Work out the finished part from the listing and answer in its coordinate system (mm). A direction names the side the tool comes from. Coordinates: 2 decimals unless noted, no trailing zeros. Order: outer loops, then holes, each group sorted by start corner. A loop starts at its lowest first (then second) coordinate and runs counter-clockwise, first axis right, second up.
1. The part is cut by section B-B, the plane y = 61.5. Give the vertices of the cut face in (x, z), then the cut area to 4 significant figures.
2. Determine the mould class of faces 1 (the cylindrical face through (-79.446, -137.712, 2.465)), 2 (the cylindrical face through (123.956, 0.266, 2.465)), 3 (the cylindrical face through (146.99, 97.15, 2.54)) for opening direction Y: +Y half, -Y half, draft (parallel to the pull), parting line (faces both ways), or undercut.
3. Flat-ended cylindrical pins translate along their axes: pin 1 Ø5 at (x, y) = (192.5, -100) entering from +Z; pin 2 Ø1 at (y, z) = (-7, 2.5) entering from -X; pin 3 Ø2 at (x, z) = (143.5, 2) entering from +Y. Find the tip coordinate at first contact, or state that the pin passes through.
4. The part is cut by section D-D, the plane z = 1.4. Count the separate pieces of the cut face and the enclosed holes in it, then the cut area to 3 significant figures.
5. The part is cut by section A-A, the plane x = 50. Give the vertices of the cut face in (y, z), then the cut area to 4 significant figures.
6. The part is cut by section C-C, the plane x = 130. Give the vertices of the cut face in (y, z).
7. Find the intervals of material crossed by probe 1 along Y at (x, z) = (14, 2.65); probe 2 along Y at (x, z) = (178.5, 0.8); probe 3 along X at (y, z) = (-73.5, 4.75), in increasing order.
8. A tool of negligible diameter and unlimited length cuts with its end or side. For faces 4 (the cylindrical face through (-147.15, 96.99, 2.54)), 5 (the cylindrical face through (79.055, -136.97, 2.465)), 6 (the flat face through (-78, -44, 3)), from which of +Z, -Z, +X, -X, +Y, -Y can it reach the whole face along a straight path? Write none if from no direction.
```python
from build123d import *

# Parameters (mm, degrees)
EXTRUDE_1_OUTLINE_R   = 2
EXTRUDE_1_OUTLINE_R_2 = 6.05
EXTRUDE_1_DEPTH       = 5
CUT_EXTRUDE_START     = -2
SKETCH_2_R            = 3
SKETCH_2_R_2          = 2
CUT_EXTRUDE_1_DEPTH   = 2
SKETCH_3_R            = 31
SKETCH_3_R_2          = 32
CUT_EXTRUDE_2_DEPTH   = 281.579587951
FILLET_1_R            = 10
SKETCH1_R             = 11.937888281
CUT_EXTRUDE1_DEPTH    = 10
FILLET1_R             = 5


# Read off the part's stored shape, not the designer's step: 凸台-拉伸1
with BuildPart() as part:
    # 凸台-拉伸1 outline → 凸台-拉伸1 (new body)
    with BuildSketch(Plane.XY):
        with BuildLine():
            ThreePointArc((-97.800454043, -160.623488863), (-77.281489026, -133.346936317), (-70, -100))
            Line((-70, -100), (70, -100))
            ThreePointArc((70, -100), (77.281489026, -133.346936317), (97.800454043, -160.623488863))
            Line((97.800454043, -160.623488863), (202.199545957, -160.623488863))
            ThreePointArc((202.199545957, -160.623488863), (224.999597029, -72.160092574), (150, -20))
            Line((150, -20), (150, 100))
            Line((150, 100), (-150, 100))
            Line((-150, 100), (-150, -20))
            ThreePointArc((-150, -20), (-224.999597029, -72.160092574), (-202.199545957, -160.623488863))
            Line((-202.199545957, -160.623488863), (-97.800454043, -160.623488863))
        make_face()
        with Locations((-180.0520382, -130.0520382)):
            Circle(EXTRUDE_1_OUTLINE_R, mode=Mode.SUBTRACT)
        with Locations((-150, -142.5)):
            Circle(EXTRUDE_1_OUTLINE_R, mode=Mode.SUBTRACT)
        with Locations((-119.9479618, -130.0520382)):
            Circle(EXTRUDE_1_OUTLINE_R, mode=Mode.SUBTRACT)
        with Locations((-192.5, -100)):
            Circle(EXTRUDE_1_OUTLINE_R, mode=Mode.SUBTRACT)
        with Locations((-107.5, -100)):
            Circle(EXTRUDE_1_OUTLINE_R, mode=Mode.SUBTRACT)
        with Locations((-180.0520382, -69.9479618)):
            Circle(EXTRUDE_1_OUTLINE_R, mode=Mode.SUBTRACT)
        with Locations((-119.9479618, -69.9479618)):
            Circle(EXTRUDE_1_OUTLINE_R, mode=Mode.SUBTRACT)
        with Locations((-150, -57.5)):
            Circle(EXTRUDE_1_OUTLINE_R, mode=Mode.SUBTRACT)
        with Locations((-50, -80)):
            Circle(EXTRUDE_1_OUTLINE_R_2, mode=Mode.SUBTRACT)
        with Locations((107.5, -100)):
            Circle(EXTRUDE_1_OUTLINE_R, mode=Mode.SUBTRACT)
        with Locations((119.9479618, -130.0520382)):
            Circle(EXTRUDE_1_OUTLINE_R, mode=Mode.SUBTRACT)
        with Locations((150, -142.5)):
            Circle(EXTRUDE_1_OUTLINE_R, mode=Mode.SUBTRACT)
        with Locations((180.0520382, -130.0520382)):
            Circle(EXTRUDE_1_OUTLINE_R, mode=Mode.SUBTRACT)
        with Locations((192.5, -100)):
            Circle(EXTRUDE_1_OUTLINE_R, mode=Mode.SUBTRACT)
        with Locations((50, -80)):
            Circle(EXTRUDE_1_OUTLINE_R_2, mode=Mode.SUBTRACT)
        with Locations((119.9479618, -69.9479618)):
            Circle(EXTRUDE_1_OUTLINE_R, mode=Mode.SUBTRACT)
        with Locations((180.0520382, -69.9479618)):
            Circle(EXTRUDE_1_OUTLINE_R, mode=Mode.SUBTRACT)
        with Locations((150, -57.5)):
            Circle(EXTRUDE_1_OUTLINE_R, mode=Mode.SUBTRACT)
        with Locations((-130, 0)):
            Circle(EXTRUDE_1_OUTLINE_R_2, mode=Mode.SUBTRACT)
        with Locations((-130, 79.62392947)):
            Circle(EXTRUDE_1_OUTLINE_R_2, mode=Mode.SUBTRACT)
        with Locations((130, 0)):
            Circle(EXTRUDE_1_OUTLINE_R_2, mode=Mode.SUBTRACT)
        with Locations((130, 80)):
            Circle(EXTRUDE_1_OUTLINE_R_2, mode=Mode.SUBTRACT)
    extrude(amount=EXTRUDE_1_DEPTH)

    # 草图2 → 切除-拉伸1 (cut)
    # profile 1 of 16: a face of its own
    with BuildSketch(Plane.XY.offset(5).offset(CUT_EXTRUDE_START)):
        with Locations((-192.5, -100)):
            Circle(SKETCH_2_R)
        with Locations((-192.5, -100)):
            Circle(SKETCH_2_R_2, mode=Mode.SUBTRACT)
    # profile 2 of 16: a face of its own
    with BuildSketch(Plane.XY.offset(5).offset(CUT_EXTRUDE_START)):
        with Locations((-180.0520382, -130.0520382)):
            Circle(SKETCH_2_R)
        with Locations((-180.0520382, -130.0520382)):
            Circle(SKETCH_2_R_2, mode=Mode.SUBTRACT)
    # profile 3 of 16: a face of its own
    with BuildSketch(Plane.XY.offset(5).offset(CUT_EXTRUDE_START)):
        with Locations((-150, -142.5)):
            Circle(SKETCH_2_R)
        with Locations((-150, -142.5)):
            Circle(SKETCH_2_R_2, mode=Mode.SUBTRACT)
    # profile 4 of 16: a face of its own
    with BuildSketch(Plane.XY.offset(5).offset(CUT_EXTRUDE_START)):
        with Locations((-119.9479618, -130.0520382)):
            Circle(SKETCH_2_R)
        with Locations((-119.9479618, -130.0520382)):
            Circle(SKETCH_2_R_2, mode=Mode.SUBTRACT)
    # profile 5 of 16: a face of its own
    with BuildSketch(Plane.XY.offset(5).offset(CUT_EXTRUDE_START)):
        with Locations((-107.5, -100)):
            Circle(SKETCH_2_R)
        with Locations((-107.5, -100)):
            Circle(SKETCH_2_R_2, mode=Mode.SUBTRACT)
    # profile 6 of 16: a face of its own
    with BuildSketch(Plane.XY.offset(5).offset(CUT_EXTRUDE_START)):
        with Locations((150, -57.5)):
            Circle(SKETCH_2_R)
        with Locations((150, -57.5)):
            Circle(SKETCH_2_R_2, mode=Mode.SUBTRACT)
    # profile 7 of 16: a face of its own
    with BuildSketch(Plane.XY.offset(5).offset(CUT_EXTRUDE_START)):
        with Locations((180.0520382, -69.9479618)):
            Circle(SKETCH_2_R)
        with Locations((180.0520382, -69.9479618)):
            Circle(SKETCH_2_R_2, mode=Mode.SUBTRACT)
    # profile 8 of 16: a face of its own
    with BuildSketch(Plane.XY.offset(5).offset(CUT_EXTRUDE_START)):
        with Locations((119.9479618, -69.9479618)):
            Circle(SKETCH_2_R)
        with Locations((119.9479618, -69.9479618)):
            Circle(SKETCH_2_R_2, mode=Mode.SUBTRACT)
    # profile 9 of 16: a face of its own
    with BuildSketch(Plane.XY.offset(5).offset(CUT_EXTRUDE_START)):
        with Locations((107.5, -100)):
            Circle(SKETCH_2_R)
        with Locations((107.5, -100)):
            Circle(SKETCH_2_R_2, mode=Mode.SUBTRACT)
    # profile 10 of 16: a face of its own
    with BuildSketch(Plane.XY.offset(5).offset(CUT_EXTRUDE_START)):
        with Locations((150, -142.5)):
            Circle(SKETCH_2_R)
        with Locations((150, -142.5)):
            Circle(SKETCH_2_R_2, mode=Mode.SUBTRACT)
    # profile 11 of 16: a face of its own
    with BuildSketch(Plane.XY.offset(5).offset(CUT_EXTRUDE_START)):
        with Locations((180.0520382, -130.0520382)):
            Circle(SKETCH_2_R)
        with Locations((180.0520382, -130.0520382)):
            Circle(SKETCH_2_R_2, mode=Mode.SUBTRACT)
    # profile 12 of 16: a face of its own
    with BuildSketch(Plane.XY.offset(5).offset(CUT_EXTRUDE_START)):
        with Locations((-150, -57.5)):
            Circle(SKETCH_2_R)
    # profile 13 of 16: a face of its own
    with BuildSketch(Plane.XY.offset(5).offset(CUT_EXTRUDE_START)):
        with Locations((-119.9479618, -69.9479618)):
            Circle(SKETCH_2_R)
    # profile 14 of 16: a face of its own
    with BuildSketch(Plane.XY.offset(5).offset(CUT_EXTRUDE_START)):
        with Locations((-180.0520382, -69.9479618)):
            Circle(SKETCH_2_R)
    # profile 15 of 16: a face of its own
    with BuildSketch(Plane.XY.offset(5).offset(CUT_EXTRUDE_START)):
        with Locations((119.9479618, -130.0520382)):
            Circle(SKETCH_2_R)
    # profile 16 of 16: a face of its own
    with BuildSketch(Plane.XY.offset(5).offset(CUT_EXTRUDE_START)):
        with Locations((192.5, -100)):
            Circle(SKETCH_2_R)
    extrude(amount=CUT_EXTRUDE_1_DEPTH, mode=Mode.SUBTRACT)

    # 草图3 → 切除-拉伸2 (cut, through all)
    with BuildSketch(Plane.XY.offset(5)):
        with Locations((-150, -100)):
            Circle(SKETCH_3_R)
        with Locations((150, -100)):
            Circle(SKETCH_3_R_2)
    extrude(amount=-CUT_EXTRUDE_2_DEPTH, mode=Mode.SUBTRACT)

    # 圆角1
    fillet_1_edges = [part.edges().sort_by_distance(p)[0] for p in [
        (-150, -20, 2.5),
        (-150, 100, 2.5),
        (150, 100, 2.5),
        (150, -20, 2.5),
        (70, -100, 2.5),
        (-70, -100, 2.5),
    ]]
    fillet(fillet_1_edges, radius=FILLET_1_R)

    # Sketch1 → Cut-Extrude1 (cut)
    # profile 1 of 6: a face of its own
    with BuildSketch(Plane.XY.offset(5)):
        Polygon((-90, 70), (-40, 50), (40, 50), (90, 70), (60, 85), (-60, 85), align=None)
    # profile 2 of 6: a face of its own
    with BuildSketch(Plane.XY.offset(5)):
        Polygon((-110, 50), (-110, 20), (-50, 30), align=None)
    # profile 3 of 6: a face of its own
    with BuildSketch(Plane.XY.offset(5)):
        Polygon((50, 30), (110, 20), (110, 50), align=None)
    # profile 4 of 6: a face of its own
    with BuildSketch(Plane.XY.offset(5)):
        Polygon((-25, 30), (25, 30), (20, -80), (-20, -80), align=None)
        Circle(SKETCH1_R, mode=Mode.SUBTRACT)
    # profile 5 of 6: a face of its own
    with BuildSketch(Plane.XY.offset(5)):
        Polygon((-90, 0), (-50, -30), (-110, -60), align=None)
    # profile 6 of 6: a face of its own
    with BuildSketch(Plane.XY.offset(5)):
        Polygon((50, -30), (90, 0), (110, -60), align=None)
    extrude(amount=-CUT_EXTRUDE1_DEPTH, mode=Mode.SUBTRACT)


with BuildPart() as body_2:
    # of the pieces the cut leaves, the one that is kept (cut_extrude1_keep)
    add(part.part.solids().sort_by_distance((-158.888888889, -20.4953608, 0))[0])

    # Fillet1
    fillet1_edges = [body_2.edges().sort_by_distance(p)[0] for p in [
        (-60, 85, 2.5),
        (60, 85, 2.5),
        (90, 70, 2.5),
        (40, 50, 2.5),
        (-40, 50, 2.5),
        (-90, 70, 2.5),
        (50, -30, 2.5),
        (90, 0, 2.5),
        (110, -60, 2.5),
        (-25, 30, 2.5),
        (25, 30, 2.5),
        (20, -80, 2.5),
        (-20, -80, 2.5),
        (-50, 30, 2.5),
        (-110, 20, 2.5),
        (-110, 50, 2.5),
        (110, 50, 2.5),
        (110, 20, 2.5),
        (50, 30, 2.5),
        (-90, 0, 2.5),
        (-50, -30, 2.5),
        (-110, -60, 2.5),
    ]]
    fillet(fillet1_edges, radius=FILLET1_R)


solid = body_2.part
```
Geometry says:
1. outline: (-150, 0) - (-68.75, 0) - (-68.75, 5) - (-150, 5) - close; (68.75, 0) - (150, 0) - (150, 5) - (68.75, 5) - close
1. area: 812.5 mm2
2. face 1: -Y half
2. face 2: undercut
2. face 3: +Y half
3. pin 1: stops at z = 3
3. pin 2: stops at x = -150
3. pin 3: stops at y = 99.68
4. separate pieces: 1
4. enclosed holes: 30
4. area: 66,100 mm2
5. outline: (-100, 0) - (-86.05, 0) - (-86.05, 5) - (-100, 5) - close; (-73.95, 0) - (54, 0) - (54, 5) - (-73.95, 5) - close; (85, 0) - (100, 0) - (100, 5) - (85, 5) - close
5. area: 784.5 mm2
6. outline: (-160.62, 0) - (-124.98, 0) - (-124.98, 5) - (-160.62, 5) - close; (-75.02, 0) - (-6.05, 0) - (-6.05, 5) - (-75.02, 5) - close; (6.05, 0) - (73.95, 0) - (73.95, 5) - (6.05, 5) - close; (86.05, 0) - (100, 0) - (100, 5) - (86.05, 5) - close
7. probe 1: y = -100 to -80, 30 to 50, 85 to 100
7. probe 2: y = -160.62 to -131.31, -128.79 to -114.55, -85.45 to -71.21, -68.69 to -25.25
7. probe 3: x = -225.48 to -166.09, -133.91 to -20.3, 20.3 to 132.06, 167.94 to 225.48
8. face 4: +Z, -Z, -X, +Y
8. face 5: +Z, -Z, -Y
8. face 6: +Z, -Z
